For this review, take the finished solid that the model builds, in its own axes (mm). Face numbers are marked on the shaded views. A direction names the side the tool comes from. Give positions to 0.01 mm unless a question says otherwise; leave off trailing zeros. Loops run counter-clockwise (first coordinate to the right, second up) from the corner with the lowest first, then second, coordinate; pieces in that order, holes last. Notation, with made-up numbers: M -37,39 L -13,39 A19 ccw -13,76 Z; hole C -6.75,-2 d7. An arc over 180 degrees is marked long. Use CSV: the item, a comma, the result in double quotes. Start each with the question number.
1. Take a section at C-C, the plane y = 8. Write out the cut boundary in (x, z).
2. Take a section at D-D, the plane y = 13.5. Write out the cut boundary in (x, z).
3. Insertion check: P1, Ø5, axis at x = 0, z = 0, coming from the +Y side; P2, Ø6, axis at x = 9.5, y = 12.5, coming from the +Z side; P3, Ø1.5, axis at x = 0.5, y = 15, coming from the -Z side. Each pin has a flat end and moves straight along its axis. Give the tip position at first contact, or say it passes through.
4. Take a section at B-B, the plane x = 0. Write out the cut boundary in (y, z).
5. To check wall thickness, follow line 1 (X direction, y = 11.25, z = 0); line 2 (X direction, y = 6.5, z = -0.5); line 3 (Z direction, x = 4, y = 5.75). State the ranges of each line that lie inside material, in increasing order. Write a range as [from, to].
6. Tool access review of the marked faces 1 and 2: name each direction out of +Z, -Z, +X, -X, +Y, -Y from which nothing blocks a thin tool from reaching the whole face with its end or side.
7. Take a section at A-A, the plane z = 0. Write out the cut boundary in (x, y), and give its area (3 significant figures).
8. The part is to be moulded in two halves that separate along Z. For the marked faces 3, 4 and 5, say which applies: pulls with the +Z half, pulls with the -Z half, needs draft (parallel to the pull), parting line crosses it, or undercut.
from build123d import *

# Parameters (mm, degrees)
SKETCH_1_R          = 27.5
EXTRUDE_1_DEPTH     = 17
FILLET_1_R          = 5
SKETCH_2_R          = 1.5
CUT_EXTRUDE_1_DEPTH = 43.444080989
SKETCH_3_R          = 10
CUT_EXTRUDE_2_DEPTH = 2
CUT_EXTRUDE_START   = -2
SKETCH_4_R          = 10
CUT_EXTRUDE_3_DEPTH = 2
FILLET_2_R          = 3


with BuildPart() as part:
    # 草图1 → 凸台-拉伸1 (new body)
    with BuildSketch(Plane(origin=(0, 0, 0), x_dir=(1, 0, 0), z_dir=(0, 1, 0))):
        with Locations(Location((0, 0, 0), (0, 0, 270))):
            Circle(SKETCH_1_R)
    extrude(amount=EXTRUDE_1_DEPTH)

    # 圆角1
    fillet_1_edges = [part.edges().sort_by_distance(p)[0] for p in [
        (0, 0, -27.5),
        (0, 17, -27.5),
    ]]
    fillet(fillet_1_edges, radius=FILLET_1_R)

    # 草图2 → 切除-拉伸1 (cut, through all)
    with BuildSketch(Plane.XZ):
        with Locations(Location((0, 0, 0), (0, 0, 270))):
            Circle(SKETCH_2_R)
    extrude(amount=-CUT_EXTRUDE_1_DEPTH, mode=Mode.SUBTRACT)

    # 草图3 → 切除-拉伸2 (cut)
    with BuildSketch(Plane(origin=(0, 17, 0), x_dir=(1, 0, 0), z_dir=(0, 1, 0))):
        with Locations(Location((0, 0, 0), (0, 0, 270))):
            Circle(SKETCH_3_R)
    extrude(amount=-CUT_EXTRUDE_2_DEPTH, mode=Mode.SUBTRACT)

    # 草图4 → 切除-拉伸3 (cut)
    with BuildSketch(Plane.XZ.offset(CUT_EXTRUDE_START)):
        with Locations(Location((0, 0, 0), (0, 0, 90))):
            Circle(SKETCH_4_R)
    extrude(amount=CUT_EXTRUDE_3_DEPTH, mode=Mode.SUBTRACT)

    # 圆角2
    # the kernel refuses this fillet: 3 mm, written as the material it adds along each edge
    with BuildSketch(Plane(origin=(0, 15, 0), x_dir=(0, 0, 1), z_dir=(-1, 0, 0))) as fillet_2_piece_1:
        with BuildLine():
            CenterArc((7.171572875, 3), FILLET_2_R, 270, 70.528779366)
            Line((7.171572875, 0), (7.171572875, -0.06))
            Line((7.171572875, -0.06), (10, -0.06))
            Line((10, -0.06), (10.06, 0))
            ThreePointArc((10.06, 0), (10.06, 1), (10.056568542, 1.98))
            Line((10.056568542, 1.98), (10, 2))
        make_face()
    revolve(axis=Axis((0, 15, 0), (0, 1, 0)))
    with BuildSketch(Plane(origin=(0, 2, 0), x_dir=(0, 0, 1), z_dir=(1, 0, 0))) as fillet_2_piece_2:
        with BuildLine():
            CenterArc((7.171572875, 3), FILLET_2_R, 270, 70.528779366)
            Line((7.171572875, 0), (7.171572875, -0.06))
            Line((7.171572875, -0.06), (10, -0.06))
            Line((10, -0.06), (10.06, 0))
            ThreePointArc((10.06, 0), (10.06, 1), (10.056568542, 1.98))
            Line((10.056568542, 1.98), (10, 2))
        make_face()
    revolve(axis=Axis((0, 2, 0), (0, -1, 0)))


solid = part.part
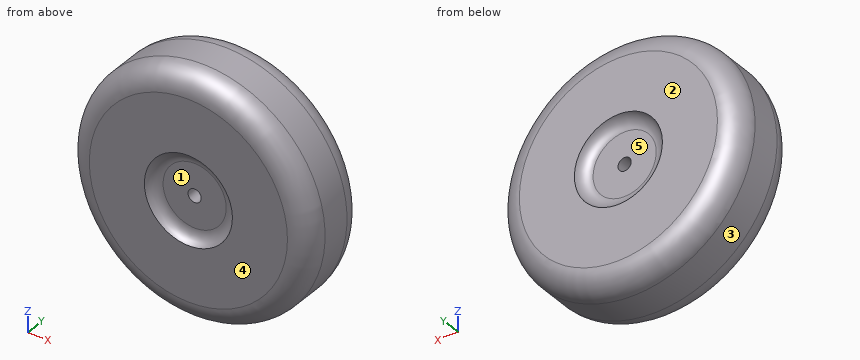
Result set:
1,outline,"C 0,0 d55; hole C 0,0 d3"
2,outline,"C 0,0 d54.54; hole C 0,0 d3"
3,P1,"y = 15"
3,P2,"z = 26.71"
3,P3,"z = -26.96"
4,outline,"M 0,-22.5 A5 ccw 5,-27.5 L 12,-27.5 A5 ccw 17,-22.5 L 17,-10 A3 cw 15,-7.17 L 15,-1.5 L 2,-1.5 L 2,-7.17 A3 cw 0,-10 Z; M 0,10 A3 cw 2,7.17 L 2,1.5 L 15,1.5 L 15,7.17 A3 cw 17,10 L 17,22.5 A5 ccw 12,27.5 L 5,27.5 A5 ccw 0,22.5 Z"
5,line 1,"[-27.5, -1.5], [1.5, 27.5]"
5,line 2,"[-27.5, -1.41], [1.41, 27.5]"
5,line 3,"[-27.21, 27.21]"
6,face 1,"-Y"
6,face 2,"+Z, -Z, +X, -X, +Y"
7,outline,"M -27.5,5 A5 ccw -22.5,0 L -10,0 A3 cw -7.17,2 L -1.5,2 L -1.5,15 L -7.17,15 A3 cw -10,17 L -22.5,17 A5 ccw -27.5,12 Z; M 1.5,2 L 7.17,2 A3 cw 10,0 L 22.5,0 A5 ccw 27.5,5 L 27.5,12 A5 ccw 22.5,17 L 10,17 A3 cw 7.17,15 L 1.5,15 Z"
7,area,"801 mm2"
8,face 3,"parting line crosses it"
8,face 4,"needs draft"
8,face 5,"undercut"
